Source: CAD feature listing. Evaluate the final solid. Frame: model axes, mm. A direction names the side the tool comes from. Round coordinates to 2 decimals unless told otherwise and drop trailing zeros. Loops run counter-clockwise (first coordinate to the right, second up) from the corner with the lowest first, then second, coordinate; pieces in that order, holes last.
(1) Section B-B, the plane z = -2.5. Return the cut outline in (x, y).
(2) Mould query, pull axis Y, two halves, no side actions, for faces 4 (the cylindrical face through (-0.33, -20.52, 1.97)), 5 (the cylindrical face through (0, -19, 5)), 6 (the flat face through (2, -25, 4)). Classes: pulls with the +Y half, pulls with the -Y half, needs draft (parallel to the pull), parting line crosses it, or undercut.
(3) Material intervals for probe 1 along Y at (x, z) = (0, 2.8); probe 2 along X at (y, z) = (0.5, -2.75); probe 3 along Z at (x, y) = (-18, -4), sorted ascending.
(4) Section A-A, the plane y = 0. Count the separate pieces of the cut face and the enclosed holes in it, plus the area to 3 significant figures.
(5) First-contact query: pin 1 Ø4 at (x, y) = (19.5, 10) entering from -Z; pin 2 Ø6.5 at (x, y) = (-23, 0) entering from +Z; pin 3 Ø8 at (x, z) = (-14, -2) entering from -Y. Flat tips, straight axial feed; report the tip coordinate or a pass-through.
(6) Set-up query: faces 1 (the flat face through (4, 25, 5)), 2 (the cylindrical face through (-19, 0, 5)), 3 (the flat face through (4, -25, 5)). Return all of +Z, -Z, +X, -X, +Y, -Y with unobstructed straight access to the full face (end or side cutting, diameter ignored); none if empty.
```python
from build123d import *

# Parameters (mm, degrees)
FILLET1_R               = 3
CHAMFER1_SIZE           = 0.5
CUT_EXTRUDE2_START      = -3
CUT_EXTRUDE2_DEPTH      = 3
CUT_EXTRUDE3_DEPTH      = 43.343830719
CUT_EXTRUDE3_DEPTH_BACK = 43.343830719
SKETCH3_4_R             = 2.5


# Read off the part's stored shape, not the designer's step: Cut-Extrude2
with BuildPart() as part:
    # Sketch2 → Revolve1 (revolve)
    with BuildSketch(Plane(origin=(0, 0, 0), x_dir=(-1, 0, 0), z_dir=(0, 1, 0)), mode=Mode.PRIVATE) as revolve1_sk:
        Polygon((13.5, 7), (28, 7), (28, 0), (18, 0), (18, -8), (10, -8), (10, 5), (13.5, 5), align=None)
    revolve(revolve1_sk.sketch.rotate(Axis((0, 0, 28.029292285), (0, 0, -1)), 180), axis=Axis((0, 0, 28.029292285), (0, 0, -1)))

    # Fillet1
    fillet1_edges = [part.edges().sort_by_distance(p)[0] for p in [
        (-28, 0, 7),
    ]]
    fillet(fillet1_edges, radius=FILLET1_R)

    # Chamfer1
    chamfer1_edges = [part.edges().sort_by_distance(p)[0] for p in [
        (-10, 0, 5),
    ]]
    chamfer(chamfer1_edges, length=CHAMFER1_SIZE)

    # Cut-Extrude2 outline → Cut-Extrude2 (cut)
    with BuildSketch(Plane.XY.offset(7).offset(CUT_EXTRUDE2_START)):
        with BuildLine():
            Line((-4, 27.712812921), (-4, 23))
            ThreePointArc((-4, 23), (0, 19), (4, 23))
            Line((4, 23), (4, 27.712812921))
            ThreePointArc((4, 27.712812921), (0, 28), (-4, 27.712812921))
        make_face()
        with BuildLine():
            ThreePointArc((23, 4), (19, 0), (23, -4))
            Line((23, -4), (27.712812921, -4))
            ThreePointArc((27.712812921, -4), (28, 0), (27.712812921, 4))
            Line((27.712812921, 4), (23, 4))
        make_face()
        with BuildLine():
            ThreePointArc((4, -23), (0, -19), (-4, -23))
            Line((-4, -23), (-4, -27.712812921))
            ThreePointArc((-4, -27.712812921), (0, -28), (4, -27.712812921))
            Line((4, -27.712812921), (4, -23))
        make_face()
        with BuildLine():
            ThreePointArc((-23, -4), (-19, 0), (-23, 4))
            Line((-23, 4), (-27.712812921, 4))
            ThreePointArc((-27.712812921, 4), (-28, 0), (-27.712812921, -4))
            Line((-27.712812921, -4), (-23, -4))
        make_face()
    extrude(amount=CUT_EXTRUDE2_DEPTH, mode=Mode.SUBTRACT)

    # Sketch3_4 → Cut-Extrude3 (cut, two sides: drawn at the far end of the back side and taken through both)
    with BuildSketch(Plane.XY.offset(7).offset(-CUT_EXTRUDE3_DEPTH_BACK)):
        with Locations((0, 23)):
            Circle(SKETCH3_4_R)
        with Locations((23, 0)):
            Circle(SKETCH3_4_R)
        with Locations((0, -23)):
            Circle(SKETCH3_4_R)
        with Locations((-23, 0)):
            Circle(SKETCH3_4_R)
    extrude(amount=CUT_EXTRUDE3_DEPTH + CUT_EXTRUDE3_DEPTH_BACK, mode=Mode.SUBTRACT)


solid = part.part
```
Output values:
1. outline: circle Ø36 at (0, 0); hole circle Ø20 at (0, 0)
2. face 4: undercut
2. face 5: pulls with the -Y half
2. face 6: needs draft
3. probe 1: y = -28 to -25.5, -20.5 to -10, 10 to 20.5, 25.5 to 28
3. probe 2: x = -17.99 to -9.99, 9.99 to 17.99
3. probe 3: z = 0 to 7
4. separate pieces: 4
4. enclosed holes: 0
4. area: 272 mm2
5. pin 1: stops at z = 0
5. pin 2: stops at z = 4
5. pin 3: stops at y = -25.94
6. face 1: +Z, +Y
6. face 2: +Z, -X
6. face 3: +Z, -Y
